Can you work these out from the model? Positions are in its coordinate system, mm. Face numbers are marked on the shaded views. A direction names the side the tool comes from. Round coordinates to 2 decimals unless told otherwise and drop trailing zeros. Write each loop counter-clockwise with the first axis right and the second up, starting at its lowest first coordinate (ties: lowest second). Pieces come first, ordered by that corner, then holes.
Q1. If we section it at D-D (y = -5.75): Please give me the cut outline in (x, z).
Q2. If we section it at B-B (z = -1): Please give me the cut outline in (x, y).
Q3. If we section it at A-A (y = 5): Please give me the cut outline in (x, z), plus the area to 3 significant figures.
Q4. We'd pull the mould along Z, two halves only. Please class the marked faces 4, 5 and 6: +Z half, -Z half, draft (parallel to the pull), parting line (faces both ways), or undercut.
Q5. If we section it at C-C (x = 14): Please give me the cut outline in (y, z).
Q6. I'm going to push flat-ended pins straight in: pin 1 Ø3 at (y, z) = (-2, 3.5) entering from +X; pin 2 Ø2 at (x, y) = (-23, 4.5) entering from +Z; pin 3 Ø6.5 at (x, y) = (-24.75, 5) entering from +Z. Where does each tip first touch, or does it pass through?
Q7. Please list where these lines run through material, in increasing order: line 1 along Y through (x, z) = (-24.75, -2.3); line 2 along Y through (x, z) = (24, -1); line 3 along Y through (x, z) = (-10, -15.15) (3 decimals).
Q8. For the marked faces 1, 2 and 3, which set-ups out of +Z, -Z, +X, -X, +Y, -Y let a thin tool reach every point of the face, with its end or its side?
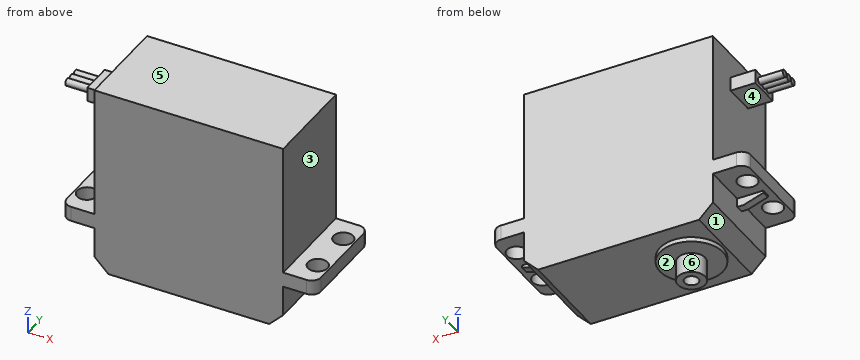
from build123d import *

# Parameters (mm, degrees)
BOSS_EXTRU_1_DEPTH                = 10.3
ESQUISSE3_W                       = 7
ESQUISSE3_H                       = 20.6
ESQUISSE3_R                       = 2.1
BOSS_EXTRU_2_DEPTH                = 3.2
BOSS_EXTRU_3_DEPTH                = 0.85
ESQUISSE8_R                       = 6.75
BOSS_EXTRU_7_DEPTH                = 1
ESQUISSE5_R                       = 2.925
BOSS_EXTRU_4_DEPTH                = 4.3
CONG_1_R                          = 2
ESQUISSE6_W                       = 3
ESQUISSE6_H                       = 6.8
BOSS_EXTRU_5_DEPTH                = 5.3
ESQUISSE7_R                       = 0.75
BOSS_EXTRU_6_DEPTH                = 5.3
DIAM_TRE_DU_PER_AGE_3_0_3_1_D     = 3
DIAM_TRE_DU_PER_AGE_3_0_3_1_DEPTH = 6
DIAM_TRE_DU_PER_AGE_3_0_3_1_TIP   = 0.901290929


with BuildPart() as part:
    # Esquisse1 → Boss.-Extru.1 (new, symmetric)
    with BuildSketch(Plane(origin=(0, 0, 0), x_dir=(1, 0, 0), z_dir=(0, 1, 0))):
        Polygon((-17.25, 12.7), (17.25, 12.7), (20.25, 9.7), (20.25, -28.2), (-20.25, -28.2), (-20.25, 9.7), align=None)
    extrude(amount=BOSS_EXTRU_1_DEPTH, both=True)

    # Esquisse3 → Boss.-Extru.2 (add)
    # profile 1 of 2: a face of its own
    with BuildSketch(Plane.XY):
        with Locations((23.75, 0)):
            Rectangle(ESQUISSE3_W, ESQUISSE3_H)
        with Locations((24.75, 5)):
            Circle(ESQUISSE3_R, mode=Mode.SUBTRACT)
        with Locations(Location((24.75, -5, 0), (0, 0, 180))):
            Circle(ESQUISSE3_R, mode=Mode.SUBTRACT)
    # profile 2 of 2: a face of its own
    with BuildSketch(Plane.XY):
        with Locations((-23.75, 0)):
            Rectangle(ESQUISSE3_W, ESQUISSE3_H)
        with Locations(Location((-24.75, 5, 0), (0, 0, 180))):
            Circle(ESQUISSE3_R, mode=Mode.SUBTRACT)
        with Locations((-24.75, -5)):
            Circle(ESQUISSE3_R, mode=Mode.SUBTRACT)
    extrude(amount=-BOSS_EXTRU_2_DEPTH)

    # Esquisse4 → Boss.-Extru.3 (add, symmetric)
    with BuildSketch(Plane(origin=(0, 0, 0), x_dir=(1, 0, 0), z_dir=(0, 1, 0))):
        Polygon((20.25, 3.2), (20.25, 5.1), (21.65, 5.1), (25.9, 3.7), (25.9, 3.2), align=None)
        Polygon((-25.9, 3.2), (-20.25, 3.2), (-20.25, 5.1), (-21.65, 5.1), (-25.9, 3.7), align=None)
    extrude(amount=BOSS_EXTRU_3_DEPTH, both=True)

    # Esquisse8 → Boss.-Extru.7 (add)
    with BuildSketch(Plane(origin=(0, 0, -12.7), x_dir=(-1, 0, 0), z_dir=(0, 0, -1))):
        with Locations(Location((10, 0, 0), (0, 0, 180))):
            Circle(ESQUISSE8_R)
    extrude(amount=BOSS_EXTRU_7_DEPTH)

    # Esquisse5 → Boss.-Extru.4 (add)
    with BuildSketch(Plane(origin=(0, 0, -13.7), x_dir=(-1, 0, 0), z_dir=(0, 0, -1))):
        with Locations(Location((10, 0, 0), (0, 0, 180))):
            Circle(ESQUISSE5_R)
    extrude(amount=BOSS_EXTRU_4_DEPTH)

    # Congé1
    cong_1_edges = [part.edges().sort_by_distance(p)[0] for p in [
        (27.25, 10.3, -1.6),
        (27.25, -10.3, -1.6),
        (-27.25, -10.3, -1.6),
        (-27.25, 10.3, -1.6),
    ]]
    fillet(cong_1_edges, radius=CONG_1_R)

    # Esquisse6 → Boss.-Extru.5 (add)
    with BuildSketch(Plane.ZY.offset(20.25)):
        with Locations((21.4, 0)):
            Rectangle(ESQUISSE6_W, ESQUISSE6_H)
    extrude(amount=BOSS_EXTRU_5_DEPTH)

    # Esquisse7 → Boss.-Extru.6 (add)
    with BuildSketch(Plane.ZY.offset(25.55)):
        with Locations((21.4, 0)):
            Circle(ESQUISSE7_R)
        with Locations((21.4, 1.6)):
            Circle(ESQUISSE7_R)
        with Locations(Location((21.4, -1.6, 0), (0, 0, 180))):
            Circle(ESQUISSE7_R)
    extrude(amount=BOSS_EXTRU_6_DEPTH)

    # Diamètre du perçage Ø3.0 (3)1
    with Locations(Plane(origin=(0, 0, -18), x_dir=(-1, 0, 0), z_dir=(0, 0, -1))):
        with Locations((10, 0)):
            Hole(DIAM_TRE_DU_PER_AGE_3_0_3_1_D / 2, depth=DIAM_TRE_DU_PER_AGE_3_0_3_1_DEPTH)
            with Locations((0, 0, -(DIAM_TRE_DU_PER_AGE_3_0_3_1_DEPTH + DIAM_TRE_DU_PER_AGE_3_0_3_1_TIP / 2))):  # 118° drill point
                Cone(0, DIAM_TRE_DU_PER_AGE_3_0_3_1_D / 2, DIAM_TRE_DU_PER_AGE_3_0_3_1_TIP, mode=Mode.SUBTRACT)


solid = part.part
A:
1. outline: (-27.25, -3.2) - (-26.71, -3.2) - (-26.71, 0) - (-27.25, 0) - close; (-22.79, -3.2) - (-20.25, -3.2) - (-20.25, -9.7) - (-17.25, -12.7) - (-13.54, -12.7) - (-13.54, -13.7) - (-6.46, -13.7) - (-6.46, -12.7) - (17.25, -12.7) - (20.25, -9.7) - (20.25, -3.2) - (22.79, -3.2) - (22.79, 0) - (20.25, 0) - (20.25, 28.2) - (-20.25, 28.2) - (-20.25, 0) - (-22.79, 0) - close; (26.71, -3.2) - (27.25, -3.2) - (27.25, 0) - (26.71, 0) - close
2. outline: (-27.25, -8.3) arc R2 ccw to (-25.25, -10.3) - (25.25, -10.3) arc R2 ccw to (27.25, -8.3) - (27.25, 8.3) arc R2 ccw to (25.25, 10.3) - (-25.25, 10.3) arc R2 ccw to (-27.25, 8.3) - close; hole circle Ø4.2 at (-24.75, -5); hole circle Ø4.2 at (-24.75, 5); hole circle Ø4.2 at (24.75, -5); hole circle Ø4.2 at (24.75, 5)
3. outline: (-27.25, -3.2) - (-26.85, -3.2) - (-26.85, 0) - (-27.25, 0) - close; (-22.65, -3.2) - (-20.25, -3.2) - (-20.25, -9.7) - (-17.25, -12.7) - (-14.53, -12.7) - (-14.53, -13.7) - (-5.47, -13.7) - (-5.47, -12.7) - (17.25, -12.7) - (20.25, -9.7) - (20.25, -3.2) - (22.65, -3.2) - (22.65, 0) - (20.25, 0) - (20.25, 28.2) - (-20.25, 28.2) - (-20.25, 0) - (-22.65, 0) - close; (26.85, -3.2) - (27.25, -3.2) - (27.25, 0) - (26.85, 0) - close
3. area: 1,670 mm2
4. face 4: undercut
4. face 5: +Z half
4. face 6: draft
5. outline: (-10.3, -12.7) - (10.3, -12.7) - (10.3, 28.2) - (-10.3, 28.2) - close
6. pin 1: stops at x = 20.25
6. pin 2: stops at z = 0
6. pin 3: stops at z = 22.9
7. line 1: y = -10.3 to -7.1, -2.9 to 2.9, 7.1 to 10.3
7. line 2: y = -10.3 to -6.96, -3.04 to 3.04, 6.96 to 10.3
7. line 3: y = -2.925 to -1.5, 1.5 to 2.925
8. face 1: -Z, -X, +Y, -Y
8. face 2: -Z
8. face 3: +Z, +X, +Y, -Y
